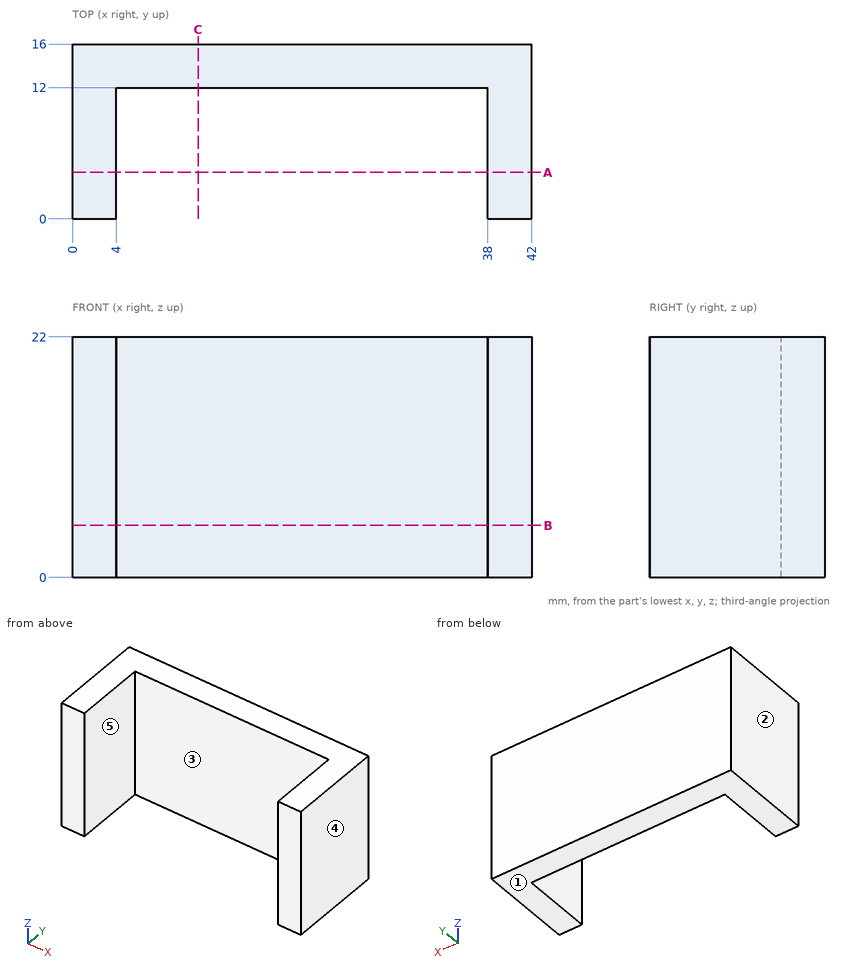
Could you check a few things on this drawing? It's one solid part, dimensions in mm from its lowest x, y, z. A direction names the side the tool comes from. Give positions to 0.01 mm unless a question says otherwise; leave off trailing zeros. Loops run counter-clockwise (first coordinate to the right, second up) from the corner with the lowest first, then second, coordinate; pieces in that order, holes last. Notation, with made-up numbers: (-34.75, 4) -> (2.25, 4) arc R6 ccw to (2.25, 8) -> close; hole circle Ø1 at (10.5, 17). An arc over 180 degrees is marked (long way). Use one line per item in the form item = value. Start each with the question number.
1) Imagine slicing it at B-B (z = 4.75). Please give me the cut outline in (x, y), then the cut area to 3 significant figures.
2) Which directions (+Z, -Z, +X, -X, +Y, -Y) give clear straight access to the entire face, cutting with the end or side of a thin tool? Please do the marked faces 4 and 5.
3) Thinking about a two-plate mould opening in X: for the marked faces 1, 2 and 3, which applies, +X half, -X half, draft (parallel to the pull), parting line (faces both ways), or undercut?
4) Please list where these lines run through material, in increasing order: line 1 along X through (y, z) = (9.5, 10.25); line 2 along Y through (x, z) = (27, 12).
5) Imagine slicing it at A-A (y = 4.25). Please give me the cut outline in (x, z).
6) Imagine slicing it at C-C (x = 11.5). Please give me the cut outline in (y, z).
Check values:
q1.outline = (0, 0) -> (4, 0) -> (4, 12) -> (38, 12) -> (38, 0) -> (42, 0) -> (42, 16) -> (0, 16) -> close
q1.area = 264 mm^2
q2.face_4 = +Z, -Z, +X, +Y, -Y
q2.face_5 = +Z, -Z, -Y
q3.face_1 = draft
q3.face_2 = -X half
q3.face_3 = undercut
q4.line_1 = 0 to 4, 38 to 42
q4.line_2 = 12 to 16
q5.outline = (0, 0) -> (4, 0) -> (4, 22) -> (0, 22) -> close; (38, 0) -> (42, 0) -> (42, 22) -> (38, 22) -> close
q6.outline = (12, 0) -> (16, 0) -> (16, 22) -> (12, 22) -> close
